Design review of the part built by this model. Coordinates are the model's own, in mm. A direction names the side the tool comes from. Give positions to 0.01 mm unless a question says otherwise; leave off trailing zeros. Loops run counter-clockwise (first coordinate to the right, second up) from the corner with the lowest first, then second, coordinate; pieces in that order, holes last. Notation, with made-up numbers: M 85.25,6.5 L 91.25,6.5 A34 cw 91.25,42.5 Z; hole C 14.25,-10 d2. An arc over 180 degrees is marked long. Use a Markdown table: item, result. Add a question column.
(1) Insertion check: pin 1 Ø3 at (x, y) = (-7, 23) entering from -Z; pin 2 Ø2.5 at (x, y) = (40, 10) entering from -Z; pin 3 Ø10 at (x, y) = (30, 9) entering from +Z; pin 4 Ø1 at (y, z) = (13, -34) entering from +X. Each pin has a flat end and moves straight along its axis. Give the tip position at first contact, or say it passes through.
(2) Add section A-A, the plane y = 10. Give the boundary of the cut face in (x, z), then the cut area to 3 significant figures.
(3) For probe 1 along Y at (x, z) = (-5, -3); probe 2 along Z at (x, y) = (12.5, 12); probe 3 along Z at (x, y) = (-2.5, 28), list the stretches that pass through material, from the lowest coordinate up.
(4) Add section B-B, the plane x = 40. Give the boundary of the cut face in (y, z), then the cut area to 3 significant figures.
(5) Draft analysis for pull direction X (two halves, no side actions). For faces 6 (the face through (-6.2, -6.2, -5)), 7 (the face through (50, 10, -85)), 8 (the face through (41.2, 9.1, -85.1)), 9 (the face through (-10, 10, -44)), state which applies: pulls with the +X half, pulls with the -X half, needs draft (parallel to the pull), parting line crosses it, or undercut.
(6) For faces 1 (the face through (-2, 0, -60)), 2 (the face through (-6.2, 23.8, -5)), 3 (the face through (-5, 10, 0)), 4 (the face through (25, 10, -80)), 5 (the face through (-5, 30, -3)), list the 3-axis set-ups (+Z, -Z, +X, -X, +Y, -Y) from which the entire face can be reached by the end or side of a thin tool; tool diameter is ignored.
(7) Add section C-C, the plane x = -5. Give the boundary of the cut face in (y, z).
(8) Add section D-D, the plane y = -5. Give the boundary of the cut face in (x, z).
```python
from build123d import *

# Parameters (mm, degrees)
Y_KSEKLIK_EKSTR_ZYON1_DEPTH      = 20
Y_KSEKLIK_EKSTR_ZYON2_DEPTH      = 10
Y_KSEKLIK_EKSTR_ZYON2_DEPTH_BACK = 30
IZIM2_W                          = 10
IZIM2_H                          = 5
IZIM3_R                          = 1.5
KES_EKSTR_ZYON1_DEPTH            = 10
IZIM4_R                          = 1.5
KES_EKSTR_ZYON2_DEPTH            = 10


with BuildPart() as part:
    # Çizim1 → Yükseklik-Ekstrüzyon1 (new body)
    with BuildSketch(Plane(origin=(0, 0, 0), x_dir=(1, 0, 0), z_dir=(0, 1, 0))):
        Polygon((-10, 0), (0, 0), (0, 80), (50, 80), (50, 90), (-10, 90), align=None)
    extrude(amount=Y_KSEKLIK_EKSTR_ZYON1_DEPTH)

    # Çizim2 → Yükseklik-Ekstrüzyon2 (add, two sides: drawn at the far end of the back side and taken through both)
    with BuildSketch(Plane(origin=(0, 20, 0), x_dir=(1, 0, 0), z_dir=(0, 1, 0)).offset(-Y_KSEKLIK_EKSTR_ZYON2_DEPTH_BACK)):
        with Locations((-5, 2.5)):
            Rectangle(IZIM2_W, IZIM2_H)
    extrude(amount=Y_KSEKLIK_EKSTR_ZYON2_DEPTH + Y_KSEKLIK_EKSTR_ZYON2_DEPTH_BACK)

    # Çizim3 → Kes-Ekstrüzyon1 (cut)
    with BuildSketch(Plane(origin=(0, 0, -5), x_dir=(-1, 0, 0), z_dir=(0, 0, -1))):
        with Locations((5, 25)):
            Circle(IZIM3_R)
        with Locations((5, -5)):
            Circle(IZIM3_R)
    extrude(amount=-KES_EKSTR_ZYON1_DEPTH, mode=Mode.SUBTRACT)

    # Çizim4 → Kes-Ekstrüzyon2 (cut)
    with BuildSketch(Plane(origin=(0, 0, -90), x_dir=(-1, 0, 0), z_dir=(0, 0, -1))):
        with Locations((-40, 10)):
            Circle(IZIM4_R)
    extrude(amount=-KES_EKSTR_ZYON2_DEPTH, mode=Mode.SUBTRACT)


solid = part.part
```
Established:
| question | item | result |
|---|---|---|
| 1 | pin 1 | z = -5 |
| 1 | pin 2 | through |
| 1 | pin 3 | z = -80 |
| 1 | pin 4 | x = 0 |
| 2 | outline | M -10,-90 L 38.5,-90 L 38.5,-80 L 0,-80 L 0,0 L -10,0 Z; M 41.5,-90 L 50,-90 L 50,-80 L 41.5,-80 Z |
| 2 | area | 1,370 mm^2 |
| 3 | probe 1 | -10 to -6.5, -3.5 to 23.5, 26.5 to 30 |
| 3 | probe 2 | -90 to -80 |
| 3 | probe 3 | -5 to 0 |
| 4 | outline | M 0,-90 L 8.5,-90 L 8.5,-80 L 0,-80 Z; M 11.5,-90 L 20,-90 L 20,-80 L 11.5,-80 Z |
| 4 | area | 170 mm^2 |
| 5 | face 6 | needs draft |
| 5 | face 7 | pulls with the +X half |
| 5 | face 8 | undercut |
| 5 | face 9 | pulls with the -X half |
| 6 | face 1 | -Z, +X, -X, -Y |
| 6 | face 2 | -Z, +X, -X, +Y |
| 6 | face 3 | +Z, +X, -X, +Y, -Y |
| 6 | face 4 | +Z, +X, +Y, -Y |
| 6 | face 5 | +Z, -Z, +X, -X, +Y |
| 7 | outline | M -10,-5 L -6.5,-5 L -6.5,0 L -10,0 Z; M -3.5,-5 L 0,-5 L 0,-90 L 20,-90 L 20,-5 L 23.5,-5 L 23.5,0 L -3.5,0 Z; M 26.5,-5 L 30,-5 L 30,0 L 26.5,0 Z |
| 8 | outline | M -10,-5 L -6.5,-5 L -6.5,0 L -10,0 Z; M -3.5,-5 L 0,-5 L 0,0 L -3.5,0 Z |
